Geometry: final body of the model. Coordinates: model frame, mm. A direction names the side the tool comes from. Give positions to 0.01 mm unless a question says otherwise; leave off trailing zeros. Loops run counter-clockwise (first coordinate to the right, second up) from the corner with the lowest first, then second, coordinate; pieces in that order, holes last. Notation, with made-up numbers: M -36.75,-28.75 L -10.75,-28.75 A36 cw -10.75,5.25 Z; hole C 51.25,43.5 d8. An arc over 180 degrees is marked long. Put each result on its own line as item: value.
```python
from build123d import *

# Parameters (mm, degrees)
AUFSATZ_LINEAR_AUSTRAGEN1_DEPTH                      = 5.5
VERRUNDUNG1_R                                        = 4
M3_GEWINDEBOHRUNG1_D                                 = 2.5
VERRUNDUNG2_R                                        = 3
SCHNITT_LINEAR_START                                 = -2
SKIZZE7_R                                            = 2.05
SCHNITT_LINEAR_AUSTRAGEN1_DEPTH                      = 23.825564349
SKIZZE7_3_R                                          = 1
SCHNITT_LINEAR_AUSTRAGEN2_DEPTH                      = 25.825564453
STIRNSENKUNG_F_R_M3_ZYLINDERSCHRAUBE_MIT_D           = 3.2
STIRNSENKUNG_F_R_M3_ZYLINDERSCHRAUBE_MIT_CBORE_D     = 6.5
STIRNSENKUNG_F_R_M3_ZYLINDERSCHRAUBE_MIT_CBORE_DEPTH = 10


with BuildPart() as part:
    # Skizze1 → Aufsatz-Linear austragen1 (new body, symmetric)
    with BuildSketch(Plane(origin=(0, 0, 0), x_dir=(1, 0, 0), z_dir=(0, 1, 0))):
        with BuildLine():
            Line((-91.978065317, 4.837587921), (-92.141327499, 0.162370724))
            Line((-92.141327499, 0.162370724), (-71.275303416, -7.43224095))
            ThreePointArc((-71.275303416, -7.43224095), (-36.187419929, -16.834010994), (0, -20))
            Line((0, -20), (0, -10))
            Line((0, -10), (-41, -10))
            Line((-41, -10), (-41, 4))
            Line((-41, 4), (-67.992685468, 4))
            Line((-67.992685468, 4), (-91.978065317, 4.837587921))
        make_face()
    extrude(amount=AUFSATZ_LINEAR_AUSTRAGEN1_DEPTH, both=True)

    # Verrundung1
    verrundung1_edges = [part.edges().sort_by_distance(p)[0] for p in [
        (-41, 0, 10),
    ]]
    fillet(verrundung1_edges, radius=VERRUNDUNG1_R)

    # M3 Gewindebohrung1 (through all)
    with Locations(Plane(origin=(-37.688737351, 5.5, 8.480848773), x_dir=(1, 0, 0), z_dir=(0, 1, 0))):
        with Locations((-7.311262649, 8.480848773)):
            Hole(M3_GEWINDEBOHRUNG1_D / 2)

    # Verrundung2
    verrundung2_edges = [part.edges().sort_by_distance(p)[0] for p in [
        (-92.141327499, 0, -0.162370724),
    ]]
    fillet(verrundung2_edges, radius=VERRUNDUNG2_R)

    # Skizze7 → Schnitt-Linear austragen1 (cut, through all)
    with BuildSketch(Plane(origin=(0.056699565, 0, -1.623663111), x_dir=(-0.999390827, 0, -0.034899497), z_dir=(0.034899497, 0, -0.999390827)).offset(SCHNITT_LINEAR_START)):
        with Locations((70.590864148, 3)):
            Circle(SKIZZE7_R)
        with Locations((89.590864148, 3)):
            Circle(SKIZZE7_R)
        with Locations((89.590864148, -3)):
            Circle(SKIZZE7_R)
        with Locations((70.590864148, -3)):
            Circle(SKIZZE7_R)
    extrude(amount=-SCHNITT_LINEAR_AUSTRAGEN1_DEPTH, mode=Mode.SUBTRACT)

    # Skizze7_3 → Schnitt-Linear austragen2 (cut, through all)
    with BuildSketch(Plane(origin=(0.056699565, 0, -1.623663111), x_dir=(-0.999390827, 0, -0.034899497), z_dir=(0.034899497, 0, -0.999390827))):
        with Locations((70.590864148, -3)):
            Circle(SKIZZE7_3_R)
        with Locations((89.590864148, -3)):
            Circle(SKIZZE7_3_R)
        with Locations((89.590864148, 3)):
            Circle(SKIZZE7_3_R)
        with Locations((70.590864148, 3)):
            Circle(SKIZZE7_3_R)
    extrude(amount=-SCHNITT_LINEAR_AUSTRAGEN2_DEPTH, mode=Mode.SUBTRACT)

    # Spiegeln3: part across plane


with BuildPart() as part_1:
    add(part.part)
    add(part.part.mirror(Plane(origin=(0, 0, 0), x_dir=(0, 0, 1), z_dir=(1, 0, 0))))

    # Stirnsenkung f_r M3 Zylinderschraube mit (through all)
    with Locations(Plane.XY.offset(20)):
        with Locations((-45, 0), (45, 0)):
            CounterBoreHole(STIRNSENKUNG_F_R_M3_ZYLINDERSCHRAUBE_MIT_D / 2, STIRNSENKUNG_F_R_M3_ZYLINDERSCHRAUBE_MIT_CBORE_D / 2, STIRNSENKUNG_F_R_M3_ZYLINDERSCHRAUBE_MIT_CBORE_DEPTH)


solid = part_1.part
```
Item 1: Set-up query: faces 1 (the flat face through (-43.6, -1.4, 10)), 2 (the cylindrical face through (-68.69, -2.91, 3.06)), 3 (the cylindrical face through (-45.74, -1.42, 2.9)). Return all of +Z, -Z, +X, -X, +Y, -Y with unobstructed straight access to the full face (end or side cutting, diameter ignored); none if empty.
Output values:
face 1: +Z
face 2: none
face 3: +Z, -Z
Item 2: Section C-C on x = 15. Output: boundary loops of the cut face in (y, z).
Output values:
outline: M -5.5,10 L 5.5,10 L 5.5,19.46 L -5.5,19.46 Z
Item 3: Pin query (flat end, axial travel): pin 1 Ø3 at (x, y) = (-45, 0) entering from +Z; pin 2 Ø6 at (x, y) = (-45, 0) entering from -Z; pin 3 Ø2 at (x, y) = (-46, 1) entering from +Z; pin 4 Ø2 at (x, y) = (-54.5, -4.5) entering from +Z. Return the tip coordinate at first contact, or that it passes through.
Output values:
pin 1: through
pin 2: z = -4
pin 3: z = 10
pin 4: z = 13.02
Item 4: Section A-A on z = 3. Count the separate pieces of the cut face and the enclosed holes in it, then the cut area to 3 significant figures.
Output values:
separate pieces: 2
enclosed holes: 6
area: 865 mm²
Item 5: Line query: probe 1 along Y at (x, z) = (-45, 5.25); probe 2 along Y at (x, z) = (45, 14.4); probe 3 along Y at (x, z) = (69.5, 2). Output: solid intervals per line, ascending. Write a range as [from, to].
Output values:
probe 1: [-5.5, -1.6], [1.6, 5.5]
probe 2: [-5.5, -3.25], [3.25, 5.5]
probe 3: [-5.5, -4.66], [-1.34, 1.34], [4.66, 5.5]
Item 6: Section D-D on x = -11. Output: boundary loops of the cut face in (y, z), then the cut area to 3 significant figures.
Output values:
outline: M -5.5,10 L 5.5,10 L 5.5,19.71 L -5.5,19.71 Z
area: 107 mm²
Item 7: Section B-B on z = 11.75. Output: boundary loops of the cut face in (x, y), then the cut area to 3 significant figures.
Output values:
outline: M -58.06,-5.5 L 58.06,-5.5 L 58.06,5.5 L -58.06,5.5 Z; hole C -45,0 d6.5; hole C 45,0 d6.5
area: 1,210 mm²
Item 8: Mould query, pull axis Z, two halves, no side actions, for faces 4 (the flat face through (-54, 0, -4)), 5 (the cylindrical face through (-68.69, 3.09, 3.06)), 6 (the flat face through (1.3, 5.5, 10.2)). Classes: pulls with the +Z half, pulls with the -Z half, needs draft (parallel to the pull), parting line crosses it, or undercut.
Output values:
face 4: pulls with the -Z half
face 5: undercut
face 6: needs draft
